The listing builds one solid part. Answer for the finished solid, in the listing's coordinates (mm). A direction names the side the tool comes from. Round coordinates to 2 decimals unless told otherwise and drop trailing zeros. Loops run counter-clockwise (first coordinate to the right, second up) from the corner with the lowest first, then second, coordinate; pieces in that order, holes last. Notation, with made-up numbers: M 4,-6 L 20,-6 A12 cw 20,10 Z; hole C 46.5,63.25 d4. An arc over 180 degrees is marked long. Answer as a JSON object with one key per item and string values.
```python
from build123d import *

# Parameters (mm, degrees)
SM_BASE_FLANGE_1_DEPTH = 30
SKETCH_4_R             = 7
SKETCH_4_R_2           = 1.5
CUT_EXTRUDE_1_DEPTH    = 10
SKETCH_5_R             = 1.5
CUT_EXTRUDE_2_DEPTH    = 10


# Sheet-metal steps are written as plain solids
with BuildPart() as part:
    # Sketch 1 → 基体-法兰1 (new body)
    with BuildSketch(Plane.XY):
        with BuildLine():
            Line((-47.024221453, 21.737024221), (-47.024221453, -8.262975779))
            ThreePointArc((-47.024221453, -8.262975779), (-46.145541797, -10.384296122), (-44.024221453, -11.262975779))
            Line((-44.024221453, -11.262975779), (-7.024221453, -11.262975779))
            Line((-7.024221453, -11.262975779), (-7.024221453, -13.262975779))
            Line((-7.024221453, -13.262975779), (-44.024221453, -13.262975779))
            ThreePointArc((-44.024221453, -13.262975779), (-47.559755359, -11.798509684), (-49.024221453, -8.262975779))
            Line((-49.024221453, -8.262975779), (-49.024221453, 21.737024221))
            Line((-49.024221453, 21.737024221), (-47.024221453, 21.737024221))
        make_face()
    extrude(amount=SM_BASE_FLANGE_1_DEPTH)

    # 草图4 → 切除-拉伸1 (cut)
    with BuildSketch(Plane.ZY.offset(49.024221453)):
        with Locations((15, 6.737024221)):
            Circle(SKETCH_4_R)
        with Locations((6.772758664, 11.487024221)):
            Circle(SKETCH_4_R_2)
        with Locations((6.772758664, 1.987024221)):
            Circle(SKETCH_4_R_2)
        with Locations((15, -2.762975779)):
            Circle(SKETCH_4_R_2)
        with Locations((23.227241336, 1.987024221)):
            Circle(SKETCH_4_R_2)
        with Locations((23.227241336, 11.487024221)):
            Circle(SKETCH_4_R_2)
        with Locations((15, 16.237024221)):
            Circle(SKETCH_4_R_2)
        with BuildLine():
            Line((30, 21.737024221), (15, 21.737024221))
            ThreePointArc((15, 21.737024221), (25.606601718, 17.343625939), (30, 6.737024221))
            Line((30, 6.737024221), (30, 21.737024221))
        make_face()
        with BuildLine():
            Line((0, 21.737024221), (0, 6.737024221))
            ThreePointArc((0, 6.737024221), (4.393398282, 17.343625939), (15, 21.737024221))
            Line((15, 21.737024221), (0, 21.737024221))
        make_face()
    extrude(amount=-CUT_EXTRUDE_1_DEPTH, mode=Mode.SUBTRACT)

    # 草图5 → 切除-拉伸2 (cut)
    with BuildSketch(Plane(origin=(0, -11.262975779, 0), x_dir=(1, 0, 0), z_dir=(0, 1, 0))):
        with Locations(Location((-38.024221453, -23, 0), (0, 0, 270))):
            Circle(SKETCH_5_R)
        with Locations(Location((-38.024221453, -7, 0), (0, 0, 270))):
            Circle(SKETCH_5_R)
        with Locations(Location((-14.024221453, -23, 0), (0, 0, 270))):
            Circle(SKETCH_5_R)
        with Locations(Location((-14.024221453, -7, 0), (0, 0, 270))):
            Circle(SKETCH_5_R)
    extrude(amount=-CUT_EXTRUDE_2_DEPTH, mode=Mode.SUBTRACT)


solid = part.part
```
Item 1: The part is cut by section B-B (z = 17). Give the vertices of the cut face in (x, y), then the cut area to 3 significant figures.
Values follow:
{"outline": "M -49.02,-8.26 A5 ccw -44.02,-13.26 L -7.02,-13.26 L -7.02,-11.26 L -44.02,-11.26 A3 cw -47.02,-8.26 L -47.02,0.03 L -49.02,0.03 Z; M -49.02,13.45 L -47.02,13.45 L -47.02,21.6 L -49.02,21.6 Z", "area": "119 mm^2"}
Item 2: Flat-ended cylindrical pins translate along their axes: P1, Ø3.5, axis at y = 11.49, z = 23.23, coming from the +X side; P2, Ø9, axis at x = -31.5, z = 21.5, coming from the +Y side. Find the tip coordinate at first contact, or state that the pin passes through.
Values follow:
{"P1": "x = -47.02", "P2": "y = -11.26"}
Item 3: Determine the mould class of faces 3 (the face through (-37.01, -12.249, 5.894)), 4 (the face through (-48.04, 2.05, 21.73)), 5 (the face through (-46.17, -10.36, 14.79)), 6 (the face through (-48.04, 11.55, 21.73)) for opening direction Y: released by +Y, released by -Y, zero draft, split by the parting line, or undercut.
Values follow:
{"face 3": "zero draft", "face 4": "undercut", "face 5": "released by +Y", "face 6": "undercut"}
Item 4: The part is cut by section A-A (z = 23). Give the vertices of the cut face in (x, y).
Values follow:
{"outline": "M -49.02,-8.26 A5 ccw -44.02,-13.26 L -39.52,-13.26 L -39.52,-11.26 L -44.02,-11.26 A3 cw -47.02,-8.26 L -47.02,0.5 L -49.02,0.5 Z; M -49.02,3.47 L -47.02,3.47 L -47.02,10 L -49.02,10 Z; M -49.02,12.97 L -47.02,12.97 L -47.02,19.43 L -49.02,19.43 Z; M -36.52,-13.26 L -15.52,-13.26 L -15.52,-11.26 L -36.52,-11.26 Z; M -12.52,-13.26 L -7.02,-13.26 L -7.02,-11.26 L -12.52,-11.26 Z"}
Item 5: Which of the six approach directions +Z, -Z, +X, -X, +Y, -Y give full straight-line access (tool end or side, diameter ignored) to faces 1 (the face through (-26, -11.263, 15)), 2 (the face through (-48.038, 14.773, 14.675))?
Values follow:
{"face 1": "+Z, -Z, +X, +Y", "face 2": "+X, -X"}
Item 6: The part is cut by section D-D (z = 2.25). Give the vertices of the cut face in (x, y), then the cut area to 3 significant figures.
Values follow:
{"outline": "M -49.02,-8.26 A5 ccw -44.02,-13.26 L -7.02,-13.26 L -7.02,-11.26 L -44.02,-11.26 A3 cw -47.02,-8.26 L -47.02,14.64 L -49.02,14.64 Z", "area": "132 mm^2"}
Item 7: The part is cut by section C-C (x = -33.5). Give the vertices of the cut face in (y, z).
Values follow:
{"outline": "M -13.26,0 L -11.26,0 L -11.26,30 L -13.26,30 Z"}
Item 8: Straight lines are drawn through the part: line 1 (Y direction, x = -48.3, z = 15); line 2 (Y direction, x = -48.6, z = 15); line 3 (X direction, y = -11.65, z = 7). For each, find the intervals that lie inside material, in ascending order.
Values follow:
{"line 1": "-10.85 to -4.26, -1.26 to -0.26, 13.74 to 14.74, 17.74 to 21.74", "line 2": "-10.28 to -4.26, -1.26 to -0.26, 13.74 to 14.74, 17.74 to 21.74", "line 3": "-47.7 to -39.52, -36.52 to -15.52, -12.52 to -7.02"}
